Could you check a few things on this model? Use its own coordinates, in mm. Face numbers are marked on the shaded views. A direction names the side the tool comes from. Round coordinates to 2 decimals unless told otherwise and drop trailing zeros. Loops run counter-clockwise (first coordinate to the right, second up) from the corner with the lowest first, then second, coordinate; pieces in that order, holes last. Notation, with made-up numbers: (31.5, -38) - (73.5, -38) arc R10 cw to (73.5, -34) - close; hole circle Ø3 at (4, -36). An arc over 180 degrees is marked (long way). Use one line per item in the form item = value.
```python
from build123d import *

# Parameters (mm, degrees)
F1_DEPTH = 10
F2_R     = 2.75
F3_DEPTH = 5.301


with BuildPart() as f1:
    # F0 (on Front) → F1 (new body, symmetric)
    with BuildSketch(Plane.XZ):
        Polygon((-10, 3.5), (-10, 0), (10, 0), (10, 3.5), (4.64, 3.5), (2.84, 5.3), (-2.84, 5.3), (-4.64, 3.5), align=None)
    extrude(amount=F1_DEPTH, both=True)

    # F2 (on face) → F3 (cut, through all)
    with BuildSketch(Plane(origin=(0, 0, 0), x_dir=(1, 0, 0), z_dir=(0, 0, -1))):
        Circle(F2_R)
    extrude(amount=-F3_DEPTH, mode=Mode.SUBTRACT)


solid = f1.part
```
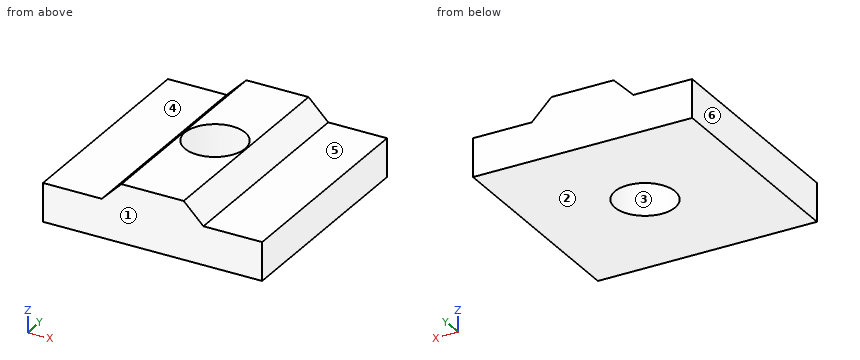
1. We'd pull the mould along Y, two halves only. Please class the marked faces 1, 2 and 3: +Y half, -Y half, draft (parallel to the pull), parting line (faces both ways), or undercut.
Solution:
face_1 = -Y half
face_2 = draft
face_3 = undercut
2. For P1, Ø6, axis at x = -8.5, y = 0.5, coming from the +Z side, with a flat end and sliding along its axis, tell me the tip position at first contact or that it passes through.
Solution:
P1 = 3.5
3. If we section it at A-A, the plane y = 0: Write out the boundary of the cut face in (x, z).
Solution:
outline = (-10, 0) - (-2.75, 0) - (-2.75, 5.3) - (-2.84, 5.3) - (-4.64, 3.5) - (-10, 3.5) - close; (2.75, 0) - (10, 0) - (10, 3.5) - (4.64, 3.5) - (2.84, 5.3) - (2.75, 5.3) - close
4. If we section it at D-D, the plane y = -5.75: Write out the boundary of the cut face in (x, z), plus the area to 3 significant figures.
Solution:
outline = (-10, 0) - (10, 0) - (10, 3.5) - (4.64, 3.5) - (2.84, 5.3) - (-2.84, 5.3) - (-4.64, 3.5) - (-10, 3.5) - close
area = 83.5 mm^2
5. If we section it at B-B, the plane x = 0: Write out the boundary of the cut face in (y, z), plus the area to 4 significant figures.
Solution:
outline = (-10, 0) - (-2.75, 0) - (-2.75, 5.3) - (-10, 5.3) - close; (2.75, 0) - (10, 0) - (10, 5.3) - (2.75, 5.3) - close
area = 76.85 mm^2
6. If we section it at C-C, the plane z = 4.45: Write out the boundary of the cut face in (x, y).
Solution:
outline = (-3.69, -10) - (3.69, -10) - (3.69, 10) - (-3.69, 10) - close; hole circle Ø5.5 at (0, 0)
7. On a 3-axis mill with a long thin cutter (end or side, diameter ignored), from which of +Z, -Z, +X, -X, +Y, -Y can I reach the whole of each face in a straight line? I mean the marked faces 4, 5 and 6. Say none if no direction works.
Solution:
face_4 = +Z, -X, +Y, -Y
face_5 = +Z, +X, +Y, -Y
face_6 = +Z, -Z, -X, +Y, -Y
8. Please list where these lines run through material, in increasing order: line 1 along Y through (x, z) = (0, 3.8); line 2 along Z through (x, y) = (8.25, -8.75).
Solution:
line_1 = -10 to -2.75, 2.75 to 10
line_2 = 0 to 3.5
